Source: CAD feature listing. Evaluate the final solid. Frame: model axes, mm. Give positions to 0.01 mm unless a question says otherwise; leave off trailing zeros. Loops run counter-clockwise (first coordinate to the right, second up) from the corner with the lowest first, then second, coordinate; pieces in that order, holes last. Notation, with made-up numbers: (65, 28.5) -> (72, 28.5) arc R18 ccw to (72, 61.5) -> close; hole circle Ø6 at (-28.75, -38). An arc over 180 degrees is marked (long way). Put each result on its own line as item: value.
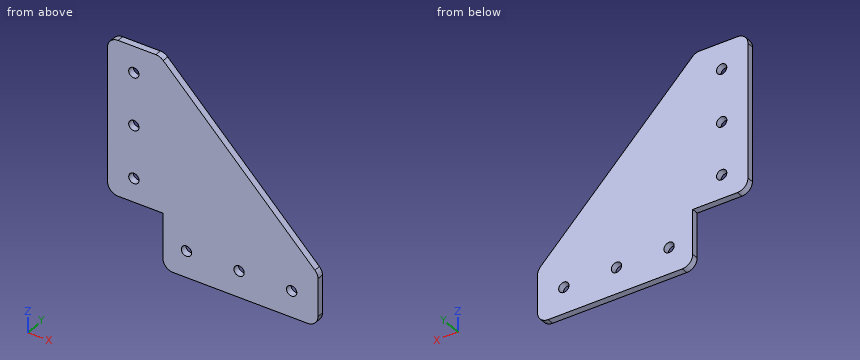
```python
from build123d import *

# Parameters (mm, degrees)
BOSS_EXTRUDE1_DEPTH = 3.175
SKETCH2_R           = 2.4892
CUT_EXTRUDE1_DEPTH  = 144.719172782
SKETCH3_W           = 26.67
SKETCH3_H           = 26.67
CUT_EXTRUDE2_DEPTH  = 144.719172782
FILLET1_R           = 5.08


with BuildPart() as part:
    # Sketch1 → Boss-Extrude1 (new body)
    with BuildSketch(Plane(origin=(0, 0, 0), x_dir=(1, 0, 0), z_dir=(0, 1, 0))):
        Polygon((0, 0), (0, 101.6), (101.6, 101.6), (101.6, 76.2), (25.4, 0), align=None)
    extrude(amount=BOSS_EXTRUDE1_DEPTH)

    # Sketch2 → Cut-Extrude1 (cut, through all)
    with BuildSketch(Plane(origin=(0, 3.175, 0), x_dir=(1, 0, 0), z_dir=(0, 1, 0))):
        with Locations(Location((12.7, 88.9, 0), (0, 0, 270))):
            Circle(SKETCH2_R)
        with Locations(Location((38.1, 88.9, 0), (0, 0, 270))):
            Circle(SKETCH2_R)
        with Locations(Location((63.5, 88.9, 0), (0, 0, 270))):
            Circle(SKETCH2_R)
        with Locations(Location((88.9, 88.9, 0), (0, 0, 270))):
            Circle(SKETCH2_R)
        with Locations(Location((12.7, 63.5, 0), (0, 0, 270))):
            Circle(SKETCH2_R)
        with Locations(Location((12.7, 38.1, 0), (0, 0, 270))):
            Circle(SKETCH2_R)
        with Locations(Location((12.7, 12.7, 0), (0, 0, 270))):
            Circle(SKETCH2_R)
    extrude(amount=-CUT_EXTRUDE1_DEPTH, mode=Mode.SUBTRACT)

    # Sketch3 → Cut-Extrude2 (cut, through all)
    with BuildSketch(Plane(origin=(0, 3.175, 0), x_dir=(1, 0, 0), z_dir=(0, 1, 0))):
        with Locations((13.335, 88.265)):
            Rectangle(SKETCH3_W, SKETCH3_H)
    extrude(amount=-CUT_EXTRUDE2_DEPTH, mode=Mode.SUBTRACT)

    # Fillet1
    fillet1_edges = [part.edges().sort_by_distance(p)[0] for p in [
        (0, 1.5875, -74.93),
        (26.67, 1.5875, -101.6),
        (0, 1.5875, 0),
        (101.6, 1.5875, -101.6),
        (101.6, 1.5875, -76.2),
        (25.4, 1.5875, 0),
    ]]
    fillet(fillet1_edges, radius=FILLET1_R)


solid = part.part
```
(1) Section B-B on x = 88.9. Return loops of the section in (y, z) (3 decimals), then the cut area to 3 significant figures.
Calculated:
outline: (0, -101.6) -> (3.175, -101.6) -> (3.175, -91.389) -> (0, -91.389) -> close; (0, -86.411) -> (3.175, -86.411) -> (3.175, -63.5) -> (0, -63.5) -> close
area: 105 mm²
(2) Section D-D on x = 12.7. Return loops of the section in (y, z) (3 decimals).
Calculated:
outline: (0, -74.93) -> (3.175, -74.93) -> (3.175, -65.989) -> (0, -65.989) -> close; (0, -61.011) -> (3.175, -61.011) -> (3.175, -40.589) -> (0, -40.589) -> close; (0, -35.611) -> (3.175, -35.611) -> (3.175, -15.189) -> (0, -15.189) -> close; (0, -10.211) -> (3.175, -10.211) -> (3.175, 0) -> (0, 0) -> close
(3) Section A-A on z = -12.7. Return loops of the section in (x, y) (3 decimals), then the cut area to 3 significant figures.
Calculated:
outline: (0, 0) -> (10.211, 0) -> (10.211, 3.175) -> (0, 3.175) -> close; (15.189, 0) -> (38.1, 0) -> (38.1, 3.175) -> (15.189, 3.175) -> close
area: 105 mm²
(4) Line query: probe 1 along X at (y, z) = (1.3, -88.9); probe 2 along X at (y, z) = (2.3, -38.1); probe 3 along X at (y, z) = (1.05, -63.5). Output: solid intervals per line, ascending. Write a range as from..to.
Calculated:
probe 1: x = 26.67..35.61, 40.59..61.01, 65.99..86.41, 91.39..101.6
probe 2: x = 0..10.21, 15.19..63.5
probe 3: x = 0..10.21, 15.19..88.9
(5) First-contact query: P1, Ø1.6, axis at y = 1, z = -90.5, coming from the -X side. Flat tip, straight axial feed; report the tip coordinate or a pass-through.
Calculated:
P1: stops at x = 26.67
(6) Section C-C on y = 2.3. Return loops of the section in (x, z), then the cut area to 3 significant figures.
Calculated:
outline: (0, -69.85) arc R5.08 ccw to (5.08, -74.93) -> (26.67, -74.93) -> (26.67, -96.52) arc R5.08 ccw to (31.75, -101.6) -> (96.52, -101.6) arc R5.08 ccw to (101.6, -96.52) -> (101.6, -78.3) arc R5.08 ccw to (100.11, -74.71) -> (26.89, -1.49) arc R5.08 ccw to (23.3, 0) -> (5.08, 0) arc R5.08 ccw to (0, -5.08) -> close; hole circle Ø4.98 at (12.7, -63.5); hole circle Ø4.98 at (12.7, -38.1); hole circle Ø4.98 at (12.7, -12.7); hole circle Ø4.98 at (38.1, -88.9); hole circle Ø4.98 at (63.5, -88.9); hole circle Ø4.98 at (88.9, -88.9)
area: 6,570 mm²
